For this review, take the finished solid that the model builds, in its own axes (mm). Coordinates: 2 decimals unless noted, no trailing zeros. Order: outer loops, then holes, each group sorted by start corner. A loop starts at its lowest first (then second) coordinate and runs counter-clockwise, first axis right, second up. Notation, with made-up numbers: M 64.25,6.25 L 102.25,6.25 A28 ccw 102.25,32.25 Z; hole C 77.5,82 d3. An arc over 180 degrees is marked long. Use one line per item in the form item = value. Start each with the question number.
```python
from build123d import *

# Parameters (mm, degrees)
F1_DEPTH       = 43.688
F2_D           = 5.5
F2_CSINK_D     = 11.2
F2_CSINK_ANGLE = 90


with BuildPart() as f1:
    # F0 (on Top) → F1 (new body)
    with BuildSketch(Plane.XY):
        with BuildLine():
            Line((-17.0035926461, 28.0065052211), (-34.7550207913, 28.0065052211))
            ThreePointArc((-34.7550207913, 28.0065052211), (-39.2451488518, 26.1466332817), (-41.1050207913, 21.6565052211))
            Line((-41.1050207913, 21.6565052211), (-41.1050207913, -27.5029422879))
            ThreePointArc((-41.1050207913, -27.5029422879), (-39.2451488518, -31.9930703485), (-34.7550207913, -33.8529422879))
            Line((-34.7550207913, -33.8529422879), (-17.0035926461, -33.8529422879))
            ThreePointArc((-17.0035926461, -33.8529422879), (-12.5134645856, -31.9930703485), (-10.6535926461, -27.5029422879))
            Line((-10.6535926461, -27.5029422879), (-10.6535926461, 21.6565052211))
            ThreePointArc((-10.6535926461, 21.6565052211), (-12.5134645856, 26.1466332817), (-17.0035926461, 28.0065052211))
        make_face()
    extrude(amount=-F1_DEPTH)

    # F2 (through all)
    with Locations(Plane.XY):
        with Locations((-25.8793067187, -2.9232185334)):
            CounterSinkHole(F2_D / 2, F2_CSINK_D / 2, counter_sink_angle=F2_CSINK_ANGLE)


solid = f1.part
```
1. For pin 1 Ø8 at (x, z) = (-15, -26.5) entering from -Y; pin 2 Ø4.5 at (x, y) = (-25.88, -2.92) entering from +Z, all flat-tipped, find the tip position at first contact; note any pin that passes through.
2. Consider section C-C, the plane x = -38. Write out the cut boundary in (y, z).
3. Consider section B-B, the plane x = -14. Write out the cut boundary in (y, z), plus the area to 3 significant figures.
4. To check wall thickness, follow line 1 (Y direction, x = -25, z = -20); line 2 (Y direction, x = -28, z = -27.5); line 3 (Y direction, x = -15, z = -28). State the ranges of each line that lie inside material, in increasing order.
5. Consider section A-A, the plane z = -37. Write out the cut boundary in (x, y).
6. The part is to be moulded in two halves that separate along X. For faces 1 (the cylindrical face through (-12.56, -32.04, -21.54)), 2 (the cylindrical face through (-39.294, -31.943, -21.538)), 3 (the cylindrical face through (-23.132, -2.802, -23.555)), 4 (the flat face through (-23, -2, -43.688)), say which applies: pulls with the +X half, pulls with the -X half, needs draft (parallel to the pull), parting line crosses it, or undercut.
Answers follow:
q1.pin_1 = -33.85
q1.pin_2 = through
q2.outline = M -32.96,-43.69 L 27.11,-43.69 L 27.11,0 L -32.96,0 Z
q3.outline = M -33.1,-43.69 L 27.25,-43.69 L 27.25,0 L -33.1,0 Z
q3.area = 2,640 mm²
q4.line_1 = -33.85 to -5.53, -0.32 to 28.01
q4.line_2 = -33.85 to -4.67, -1.17 to 28.01
q4.line_3 = -33.53 to 27.68
q5.outline = M -41.11,-27.5 A6.35 ccw -34.76,-33.85 L -17,-33.85 A6.35 ccw -10.65,-27.5 L -10.65,21.66 A6.35 ccw -17,28.01 L -34.76,28.01 A6.35 ccw -41.11,21.66 Z; hole C -25.88,-2.92 d5.5
q6.face_1 = pulls with the +X half
q6.face_2 = pulls with the -X half
q6.face_3 = undercut
q6.face_4 = needs draft
